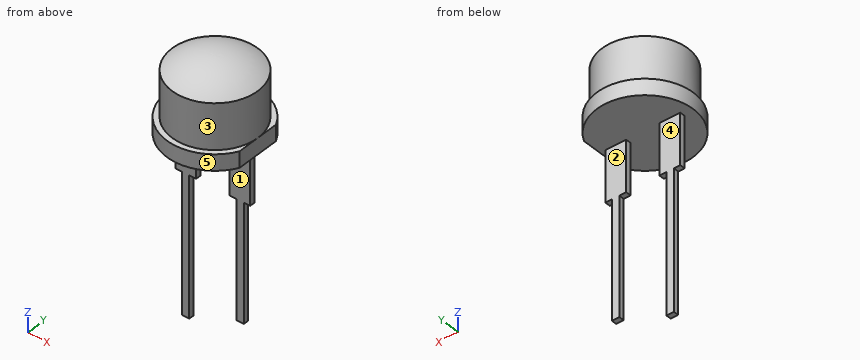
from build123d import *

# Parameters (mm, degrees)
F3_DEPTH = 7.001
F4_W     = 1.95
F4_H     = 0.5
F5_DEPTH = 4.75
F6_W     = 0.7
F6_H     = 0.5
F7_DEPTH = 11
F8_W     = 0.7
F8_H     = 0.5
F9_DEPTH = 13


with BuildPart() as f1:
    # F0 (on Front) → F1 (revolve)
    with BuildSketch(Plane.XZ):
        with BuildLine():
            Line((-4.5, 0), (0, 0))
            Line((0, 0), (0, 7))
            ThreePointArc((0, 7), (-2.096194, 6.67877), (-4, 5.744563))
            Line((-4, 5.744563), (-4, 1.5))
            Line((-4, 1.5), (-4.5, 1.5))
            Line((-4.5, 1.5), (-4.5, 0))
        make_face()
    revolve(axis=Axis((0, 0, 3.5), (0, 0, 1)))

    # F2 (on face) → F3 (cut, through all)
    with BuildSketch(Plane(origin=(0, 0, 0), x_dir=(1, 0, 0), z_dir=(0, 0, -1))):
        with BuildLine():
            ThreePointArc((4, -2.061553), (4.5, 0), (4, 2.061553))
            Line((4, 2.061553), (4, -2.061553))
        make_face()
    extrude(amount=-F3_DEPTH, mode=Mode.SUBTRACT)

    # F4 (on face) → F5 (join)
    with BuildSketch(Plane(origin=(0, 0, 0), x_dir=(1, 0, 0), z_dir=(0, 0, -1))):
        with Locations((2.525, 0)):
            Rectangle(F4_W, F4_H)
        with Locations((-2.525, 0)):
            Rectangle(F4_W, F4_H)
    extrude(amount=F5_DEPTH)

    # F6 (on face) → F7 (join)
    with BuildSketch(Plane(origin=(0, 0, -4.75), x_dir=(1, 0, 0), z_dir=(0, 0, -1))):
        with Locations((2.55, 0)):
            Rectangle(F6_W, F6_H)
    extrude(amount=F7_DEPTH)

    # F8 (on face) → F9 (join)
    with BuildSketch(Plane(origin=(0, 0, -4.75), x_dir=(1, 0, 0), z_dir=(0, 0, -1))):
        with Locations((-2.55, 0)):
            Rectangle(F8_W, F8_H)
    extrude(amount=F9_DEPTH)


with BuildPart() as f10_1:
    # F10: copy of F1
    add(f1.part)


solid = f1.part
Verification items for the finished model (mm, model axes). Face numbers are marked on the shaded views. A direction names the side the tool comes from. Coordinates: 2 decimals unless noted, no trailing zeros. Write each loop counter-clockwise with the first axis right and the second up, starting at its lowest first coordinate (ties: lowest second). Pieces come first, ordered by that corner, then holes. Notation, with made-up numbers: M 40,89 L 53,89 A7 cw 53,95 Z; hole C 68.5,44 d10. An arc over 180 degrees is marked long. One line per question, with ' | ' between items.
1) Sectioned sample at B-B on z = -15. Record the cut outline in (x, y).
Solutions:
outline: M -2.9,-0.25 L -2.2,-0.25 L -2.2,0.25 L -2.9,0.25 Z; M 2.2,-0.25 L 2.9,-0.25 L 2.9,0.25 L 2.2,0.25 Z
2) Depth check by flat-ended pin: pin 1 Ø1.5 at (x, y) = (1.5, -1.5) entering from +Z; pin 2 Ø2 at (x, y) = (-3.5, 2) entering from -Z; pin 3 Ø0.6 at (x, z) = (3, -4) entering from +Y; pin 4 Ø2.5 at (x, y) = (-1, 0) entering from +Z. Enter the tip coordinate at first touch or a pass-through.
Solutions:
pin 1: z = 6.86 | pin 2: z = 0 | pin 3: y = 0.25 | pin 4: z = 7
3) Access from +Z, -Z, +X, -X, +Y, -Y to the whole of each face (thin tool, end or side, straight path). Record for the marked faces 4 and 5.
Solutions:
face 4: -Z, +X, -X, +Y | face 5: +Z, -Z
4) Sectioned sample at C-C on z = 3.25. Record the cut outline in (x, y).
Solutions:
outline: C 0,0 d8
5) Sectioned sample at A-A on z = -4.5. Record the cut outline in (x, y).
Solutions:
outline: M -3.5,-0.25 L -1.55,-0.25 L -1.55,0.25 L -3.5,0.25 Z; M 1.55,-0.25 L 3.5,-0.25 L 3.5,0.25 L 1.55,0.25 Z
6) Release check for a two-part mould opening along Y. For the marked faces 1, 2 and 3 record: +Y half, -Y half, draft (parallel to the pull), parting line (faces both ways), or undercut.
Solutions:
face 1: -Y half | face 2: +Y half | face 3: parting line
7) Material ranges on L1, parallel to Y at x = 2.25, z = -2.5; L2, parallel to Z at x = -2, y = -3.5; L3, parallel to Z at x = 1.25, y = -3.25, recorded low to high.
Solutions:
L1: -0.25 to 0.25 | L2: 0 to 1.5 | L3: 0 to 6.07
